Autodesk Fusion 360 part; units mm, degrees
sketch "Sketch1" plane through (0, 0, 0) normal (0, 0, 1) x (1, 0, 0)
  line L0 (27.5, -10) -> (-27.5, -10)
  line L1 (-27.5, -10) -> (-27.5, 10)
  line L2 (-27.5, 10) -> (27.5, 10)
  line L3 (27.5, 10) -> (27.5, -10)
  line L4 (27.5, -10) -> (-27.5, 10) construction
  line L5 (-27.5, -10) -> (27.5, 10) construction
  line L6 (0, 0) -> (13, 0) construction
  line L7 (0, 0) -> (-13, 0) construction
  circle A0 centre (13, 0) radius 8.125
  circle A1 centre (-13, 0) radius 8.125
  line L8 (-27.5, -10) -> (27.5, -10)
  line L9 (27.5, -10) -> (27.5, -17)
  line L10 (27.5, -17) -> (-27.5, -17)
  line L11 (-27.5, -17) -> (-27.5, -10)
  line L12 (0, 10) -> (-8, 10)
  line L13 (-8, 10) -> (8, 10)
  line L14 (8, 10) -> (8, 7)
  line L15 (8, 7) -> (-8, 7)
  line L16 (-8, 7) -> (-8, 10)
  line L17 (-7, -5.75) -> (7, -5.75)
  line L18 (7, -5.75) -> (7, -14.25)
  line L19 (7, -14.25) -> (-7, -14.25)
  line L20 (-7, -14.25) -> (-7, -5.75)
  line L21 (-7, -5.75) -> (7, -14.25) construction
  line L22 (7, -5.75) -> (-7, -14.25) construction
  point P0 (0, -10)
  dimension "d1" = 55
  dimension "d2" = 20
  dimension "d3" = 13
  dimension "d4" = 13
  dimension "d5" = 16.25
  dimension "d6" = 16.25
  dimension "d7" = 7
  dimension "d8" = 8
  dimension "d9" = 16
  dimension "d10" = 3
  dimension "d11" = 14
  dimension "d12" = 8.5
extrude "Extrude1" add sketch "Sketch1" along normal blind 3 contours L0 L8 L9 L10 L11 L18 L19 L20 | L0 L1 L2 L3 L8 L14 L15 L16 L17 L18 L20
sketch "Sketch2" plane through (0, -17, 0) normal (0, -1, 0) x (1, 0, 0)
  line L0 (-27.5, 0) -> (27.5, 0)
  line L1 (27.5, 0) -> (27.5, 3)
  line L2 (27.5, 3) -> (-27.5, 3)
  line L3 (-27.5, 3) -> (-27.5, 0)
  line L4 (-27.5, 0) -> (27.5, 0)
  line L5 (27.5, 0) -> (27.5, 18)
  line L6 (27.5, 18) -> (-27.5, 18)
  line L7 (-27.5, 18) -> (-27.5, 0)
  line L8 (-27.5, 18) -> (27.5, 0) construction
  line L9 (-27.5, 0) -> (27.5, 18) construction
  line L10 (0, 9) -> (15, 9) construction
  line L11 (0, 9) -> (-15, 9) construction
  circle A0 centre (15, 9) radius 1.5
  circle A1 centre (-15, 9) radius 1.5
  dimension "d15" = 55
  dimension "d16" = 18
  dimension "d17" = 15
  dimension "d18" = 15
  dimension "d19" = 3
  dimension "d20" = 3
extrude "Extrude2" add sketch "Sketch2" along normal blind 2
sketch "Sketch3" plane through (-27.5, 0, 0) normal (-1, 0, 0) x (0, -1, 0)
  line L0 (-10, 0) -> (19, 0)
  line L1 (19, 0) -> (19, 18)
  line L2 (19, 18) -> (17, 18)
  line L3 (17, 18) -> (17, 3)
  line L4 (17, 3) -> (-10, 3)
  line L5 (-10, 3) -> (-10, 0)
  line L6 (17, 18) -> (-10, 3)
extrude "Extrude3" add sketch "Sketch3" along normal blind 0.5
sketch "Sketch4" plane through (27.5, 0, 0) normal (1, 0, 0) x (0, 1, 0)
  line L0 (-19, 0) -> (10, 0)
  line L1 (10, 0) -> (10, 3)
  line L2 (10, 3) -> (-17, 3)
  line L3 (-17, 3) -> (-17, 18)
  line L4 (-17, 18) -> (-19, 18)
  line L5 (-19, 18) -> (-19, 0)
  line L6 (-17, 18) -> (10, 3)
extrude "Extrude4" add sketch "Sketch4" along normal blind 0.5
CAD build for the part. Positions are in the model's coordinates, mm. A direction names the side the tool comes from. Round coordinates to 2 decimals unless told otherwise and drop trailing zeros. Order: outer loops, then holes, each group sorted by start corner. A loop starts at its lowest first (then second) coordinate and runs counter-clockwise, first axis right, second up. Notation, with made-up numbers: (-39.75, 0) - (-20.75, 0) arc R28 cw to (-20.75, 33) - close; hole circle Ø2 at (16.5, 18). An arc over 180 degrees is marked (long way). Return JSON: item names as keys, results as strings.
(1) Cut at D-D (z = 14.25). Give the cut face in (x, y).
Answer key:
{"outline": "(-28, -19) - (28, -19) - (28, -10.25) - (27.5, -10.25) - (27.5, -17) - (-27.5, -17) - (-27.5, -10.25) - (-28, -10.25) - close"}
(2) Cut at C-C (y = 0). Give the cut face in (x, z) (3 decimals).
Answer key:
{"outline": "(-28, 0) - (-21.125, 0) - (-21.125, 3) - (-27.5, 3) - (-27.5, 8.556) - (-28, 8.556) - close; (-4.875, 0) - (4.875, 0) - (4.875, 3) - (-4.875, 3) - close; (21.125, 0) - (28, 0) - (28, 8.556) - (27.5, 8.556) - (27.5, 3) - (21.125, 3) - close"}
(3) Cut at B-B (z = 9). Give the cut face in (x, y), then the cut area to 3 significant figures.
Answer key:
{"outline": "(-28, -19) - (-16.5, -19) - (-16.5, -17) - (-27.5, -17) - (-27.5, -0.8) - (-28, -0.8) - close; (-13.5, -19) - (13.5, -19) - (13.5, -17) - (-13.5, -17) - close; (16.5, -19) - (28, -19) - (28, -0.8) - (27.5, -0.8) - (27.5, -17) - (16.5, -17) - close", "area": "116 mm^2"}
(4) Pin check, flat tips, straight feed: pin 1 Ø2.5 at (x, z) = (-2.5, 1.5) entering from +Y; pin 2 Ø7.5 at (x, z) = (-13, 10) entering from +Y. Stop position of each tip, or through.
Answer key:
{"pin 1": "stops at y = 7", "pin 2": "stops at y = -17"}
(5) Pull direction Y, two halves, no side cores. Call faces 1 (the face through (0, -19, 9)), 2 (the face through (0, 7, 1)), 3 (the face through (4.883, -0.357, 1.479)), 4 (the face through (-16.5, -17.99, 8.93)): +Y half, -Y half, draft (parallel to the pull), parting line (faces both ways), or undercut.
Answer key:
{"face 1": "-Y half", "face 2": "+Y half", "face 3": "undercut", "face 4": "draft"}
(6) Tool access for faces 5 (the face through (0, -3, 3)), 6 (the face through (0, -18, 18)), 7 (the face through (7, -10, 1)): list every direction of +Z, -Z, +X, -X, +Y, -Y with a clear straight run to the whole face (end or side of a thin tool).
Answer key:
{"face 5": "+Z, +Y", "face 6": "+Z, +X, -X, +Y, -Y", "face 7": "+Z, -Z"}
(7) Wall check: probe 1 along Z at (x, y) = (15, -17.9); probe 2 along X at (y, z) = (-7.25, 6.25); probe 3 along Y at (x, z) = (13, 1.05) (3 decimals). Give the ranges that are in metal, low to high. Write a range as from..to.
Answer key:
{"probe 1": "z = 0..7.5, 10.5..18", "probe 2": "x = -28..-27.5, 27.5..28", "probe 3": "y = -19..-8.125, 8.125..10"}
(8) Cut at A-A (x = -1). Give the cut face in (y, z).
Answer key:
{"outline": "(-19, 0) - (-14.25, 0) - (-14.25, 3) - (-17, 3) - (-17, 18) - (-19, 18) - close; (-5.75, 0) - (7, 0) - (7, 3) - (-5.75, 3) - close"}
